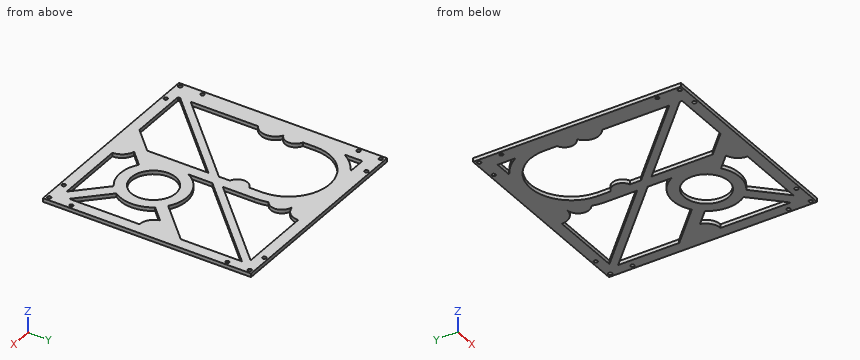
Autodesk Inventor part; units mm, degrees
ref_plane "YZ Plane" through (0, 0, 0) normal (1, 0, 0) x (0, 1, 0)
ref_plane "XZ Plane" through (0, 0, 0) normal (0, 1, 0) x (-1, 0, 0)
ref_plane "XY Plane" through (0, 0, 0) normal (0, 0, 1) x (1, 0, 0)
sketch "Sketch1" plane through (0, 0, 0) normal (0, 0, 1) x (1, 0, 0)
  line L0 (-114.3, 114.3) -> (63.5, 114.3)
  line L1 (63.5, 114.3) -> (63.5, -63.5)
  line L2 (63.5, -63.5) -> (-114.3, -63.5)
  line L3 (-114.3, -63.5) -> (-114.3, 114.3)
  circle A0 centre (6.35, -6.35) radius 19.05
  circle A1 centre (41.275, 111.125) radius 1.5875
  circle A2 centre (60.325, -41.275) radius 1.5875
  circle A3 centre (-92.075, -60.325) radius 1.5875
  circle A4 centre (-111.125, 92.075) radius 1.5875
  circle A5 centre (-111.125, 111.125) radius 1.5875
  circle A6 centre (-92.075, 111.125) radius 1.5875
  circle A7 centre (60.325, 92.075) radius 1.5875
  circle A8 centre (60.325, -60.325) radius 1.5875
  circle A9 centre (41.275, -60.325) radius 1.5875
  circle A10 centre (-111.125, -60.325) radius 1.5875
  circle A11 centre (-111.125, -41.275) radius 1.5875
  circle A12 centre (60.325, 111.125) radius 1.5875
  arc A13 (-92.7105, 44.3557) -> (-34.2895, 44.3557) centre (-63.5, 63.5) ccw construction
  line L4 (-98.425, 63.5) -> (-28.575, 63.5)
  line L5 (-28.575, 63.5) -> (-28.575, 52.7537)
  line L6 (-98.425, -53.975) -> (-98.425, -52.1151)
  line L7 (53.975, -53.975) -> (6.35, -6.35) construction
  line L8 (22.9054, -29.6406) -> (47.2398, -53.975)
  line L9 (47.2398, -53.975) -> (-12.7, -53.975)
  line L10 (6.35, -6.35) -> (40.026, 27.326) construction
  line L11 (29.6406, 10.2054) -> (41.6746, 22.2394)
  arc A14 (29.6406, -22.9054) -> (29.6406, 10.2054) centre (6.35, -6.35) ccw
  line L12 (29.6406, -22.9054) -> (53.975, -47.2398)
  line L13 (-19.05, 27.2599) -> (-19.05, 6.7409)
  arc A15 (22.9054, 16.9406) -> (-19.05, 6.7409) centre (6.35, -6.35) ccw
  line L14 (-101.6, 101.6) -> (-86.3953, 101.6)
  line L15 (-101.6, 86.3953) -> (-101.6, 101.6)
  arc A16 (-86.3953, 101.6) -> (-101.6, 86.3953) centre (-63.5, 63.5) ccw
  arc A17 (-19.05, 63.5) -> (-20.4156, 74.4333) centre (-63.5, 63.5) ccw
  line L16 (-19.05, 36.2401) -> (-19.05, 63.5)
  arc A18 (-20.4156, 74.4333) -> (-25.4, 92.075) centre (-25.4, 82.55) ccw
  arc A19 (-28.575, 52.7537) -> (-28.575, 36.1463) centre (-25.4, 44.45) ccw
  line L17 (-28.575, 36.1463) -> (-28.575, 26.7151)
  line L18 (-98.425, 52.7537) -> (-98.425, 63.5)
  arc A20 (-30.6583, 51.6182) -> (-98.425, 63.5) centre (-63.5, 63.5) ccw
  line L19 (6.35, -6.35) -> (-25.0809, -37.7809) construction
  line L20 (-10.2054, -29.6406) -> (-22.2394, -41.6746)
  arc A21 (-10.2054, -29.6406) -> (22.9054, -29.6406) centre (6.35, -6.35) ccw
  line L21 (-28.575, -34.5398) -> (-48.0102, -53.975)
  line L22 (-48.0102, -53.975) -> (-98.425, -53.975)
  line L23 (-25.0809, -37.7809) -> (-43.0414, -55.7414) construction
  line L24 (40.026, 27.326) -> (57.9865, 45.2865)
  line L25 (57.9865, 45.2865) -> (53.975, 41.275)
  arc A22 (-12.7, -53.975) -> (-22.2394, -41.6746) centre (-25.4, -53.975) ccw
  arc A23 (41.6746, 22.2394) -> (53.975, 12.7) centre (53.975, 25.4) ccw
  line L26 (53.975, 12.7) -> (53.975, -47.2398)
  arc A24 (-98.425, 14.4015) -> (-98.171, 36.2479) centre (-104.775, 25.4) ccw
  arc A25 (-98.171, 36.2479) -> (-98.425, 52.7537) centre (-101.6, 44.45) ccw
  line L27 (53.975, 48.0102) -> (53.975, 100.2849)
  line L28 (-12.7, 104.775) -> (49.4849, 104.775)
  arc A26 (-98.425, 63.5) -> (-96.3417, 51.6182) centre (-63.5, 63.5) ccw construction
  arc A27 (-25.4, 92.075) -> (-12.7, 104.775) centre (-25.4, 104.775) ccw
  line L29 (-114.3, -63.5) -> (63.5, 114.3) construction
  line L30 (-98.425, -43.1349) -> (-28.575, 26.7151)
  line L31 (-98.425, -52.1151) -> (-28.575, 17.7349)
  line L32 (22.9054, 16.9406) -> (53.975, 48.0102)
  line L33 (-19.05, 36.2401) -> (49.4849, 104.775)
  line L34 (-19.05, 27.2599) -> (53.975, 100.2849)
  line L35 (-28.575, 17.7349) -> (-28.575, -34.5398)
  line L36 (-28.575, 26.7151) -> (-28.575, 17.7349) construction
  line L37 (49.4849, 104.775) -> (53.975, 104.775) construction
  line L38 (53.975, 100.2849) -> (53.975, 104.775) construction
  line L39 (-98.425, -52.1151) -> (-98.425, -43.1349) construction
  line L40 (-98.425, -43.1349) -> (-98.425, 14.4015)
  line L41 (-25.4, -53.975) -> (-104.775, 25.4) construction
  point P0 (0, 0)
  point P1 (-101.6, 82.55)
  dimension "d0" = 114.3
  dimension "d1" = 177.8
  dimension "d2" = 177.8
  dimension "d3" = 114.3
  dimension "d4" = 38.1
  dimension "d5" = 57.15
  dimension "d6" = 57.15
  dimension "d10" = 3.175
  dimension "d11" = 3.175
  dimension "d12" = 3.175
  dimension "d15" = 3.175
  dimension "d16" = 22.225
  dimension "d17" = 22.225
  dimension "d18" = 3.175
  dimension "d19" = 3.175
  dimension "d20" = 22.225
  dimension "d23" = 3.175
  dimension "d24" = 3.175
  dimension "d25" = 22.225
  dimension "d26" = 3.175
  dimension "d27" = 3.175
  dimension "d28" = 3.175
  dimension "d29" = 3.175
  dimension "d30" = 22.225
  dimension "d34" = 3.175
  dimension "d35" = 3.175
  dimension "d36" = 3.175
  dimension "d37" = 3.175
  dimension "d38" = 22.225
  dimension "d39" = 3.175
  dimension "d40" = 3.175
  dimension "d41" = 3.175
  dimension "d42" = 3.175
  dimension "d43" = 3.175
  dimension "d44" = 3.175
  dimension "d45" = 3.175
  dimension "d46" = 22.225
  dimension "d47" = 3.175
  dimension "d48" = 3.175
  dimension "d49" = 3.175
  dimension "d50" = 3.175
  dimension "d51" = 22.225
  dimension "d52" = 3.175
  dimension "d55" = 69.85
  dimension "d56" = 50.8
  dimension "d57" = 50.8
  dimension "d93" = 69.85
  dimension "d94" = 15.875
  dimension "d97" = 38.1
  dimension "d98" = 38.1
  dimension "d99" = 38.1
  dimension "d100" = 38.1
  dimension "d101" = 19.05
  dimension "d102" = 19.05
  dimension "d103" = 19.05
  dimension "d104" = 19.05
  dimension "d212" = 9.525
  dimension "d216" = 4.7625
  dimension "d218" = 45
  dimension "d222" = 6.7352
  dimension "d226" = 28.575
  dimension "d227" = 4.7625
  dimension "d228" = 4.7625
  dimension "d232" = 9.525
extrude "Extrusion12" [suppressed]
extrude "Extrusion13" [suppressed]
hole "Hole9" [suppressed]
extrude "Extrusion14" [suppressed]
fillet "Fillet2" [suppressed]
fillet "Fillet3" [suppressed]
extrude "Extrusion15" [suppressed]
fillet "Fillet4" [suppressed]
hole "Hole10" [suppressed]
hole "Hole11" [suppressed]
hole "Hole12" [suppressed]
chamfer "Chamfer1" [suppressed]
chamfer "Chamfer2" [suppressed]
extrude "Extrusion16" [suppressed]
fillet "Fillet6" [suppressed]
extrude "Extrusion17" add sketch "Sketch1" along normal blind 3.175
properties part number "upper gearbox bottom plate"
For this review, take the finished solid that the model builds, in its own axes (mm). Give positions to 0.01 mm unless a question says otherwise; leave off trailing zeros. Loops run counter-clockwise (first coordinate to the right, second up) from the corner with the lowest first, then second, coordinate; pieces in that order, holes last.
Item 1: Take a section at B-B, the plane x = -32. State the section outline as (y, z) points (3 decimals), and give its area (3 significant figures).
Item 2: Take a section at A-A, the plane x = -83.5. State the section outline as (y, z) points (3 decimals), and give its area (3 significant figures).
Item 3: For line 1 along X through (y, z) = (57, 1.85) (3 decimals); line 2 along X through (y, z) = (50.5, 1.7) (3 decimals); line 3 along X through (y, z) = (9.5, 1.3) (3 decimals), list the stretches that pass through material, from the lowest coordinate up.
Item 4: Take a section at D-D, the plane y = -6.35. State the section outline as (x, z) points (3 decimals).
Item 5: Insertion check: pin 1 (3 mm diameter, centred on x = -111.125, y = 92.075, fed in from -Z); pin 2 (5 mm diameter, centred on x = -111.125, y = -60.325, fed in from -Z). Each pin has a flat end and moves straight along its axis. Give the tip position at first contact, or say it passes through.
Item 6: Take a section at C-C, the plane y = 40. State the section outline as (x, z) points (3 decimals).
Calculated:
1. outline: (-63.5, 0) - (-37.965, 0) - (-37.965, 3.175) - (-63.5, 3.175) - close; (14.31, 0) - (23.29, 0) - (23.29, 3.175) - (14.31, 3.175) - close; (38.494, 0) - (50.406, 0) - (50.406, 3.175) - (38.494, 3.175) - close; (78.583, 0) - (114.3, 0) - (114.3, 3.175) - (78.583, 3.175) - close
1. area: 261 mm2
2. outline: (-63.5, 0) - (-53.975, 0) - (-53.975, 3.175) - (-63.5, 3.175) - close; (-37.19, 0) - (-28.21, 0) - (-28.21, 3.175) - (-37.19, 3.175) - close; (92.131, 0) - (114.3, 0) - (114.3, 3.175) - (92.131, 3.175) - close
2. area: 129 mm2
3. line 1: x = -114.3 to -98.425, -28.575 to -19.05, 1.71 to 10.69, 53.975 to 63.5
3. line 2: x = -114.3 to -95.086, -31.914 to -19.05, -4.79 to 4.19, 53.975 to 63.5
3. line 3: x = -114.3 to -98.425, -45.79 to -36.81, -28.575 to -19.05, -17.426 to -4.218, 16.918 to 30.126, 53.975 to 63.5
4. outline: (-114.3, 0) - (-98.425, 0) - (-98.425, 3.175) - (-114.3, 3.175) - close; (-61.64, 0) - (-52.66, 0) - (-52.66, 3.175) - (-61.64, 3.175) - close; (-28.575, 0) - (-12.7, 0) - (-12.7, 3.175) - (-28.575, 3.175) - close; (25.4, 0) - (34.925, 0) - (34.925, 3.175) - (25.4, 3.175) - close; (53.975, 0) - (63.5, 0) - (63.5, 3.175) - (53.975, 3.175) - close
5. pin 1: passes through
5. pin 2: stops at z = 0
6. outline: (-114.3, 0) - (-93.904, 0) - (-93.904, 3.175) - (-114.3, 3.175) - close; (-33.096, 0) - (-19.05, 0) - (-19.05, 3.175) - (-33.096, 3.175) - close; (-15.29, 0) - (-6.31, 0) - (-6.31, 3.175) - (-15.29, 3.175) - close; (45.965, 0) - (63.5, 0) - (63.5, 3.175) - (45.965, 3.175) - close
